```python
from build123d import *

# Parameters (mm, degrees)
SKETCH1_W                        = 72.8218
SKETCH1_H                        = 66.548
BOSS_EXTRUDE1_DEPTH              = 6.35
SKETCH2_R                        = 6.35
CUT_EXTRUDE1_DEPTH               = 7.35
SKETCH3_R                        = 2.12725
CUT_EXTRUDE2_DEPTH               = 7.35
SKETCH4_R                        = 2.12725
CUT_EXTRUDE3_DEPTH               = 7.35
SKETCH5_R                        = 2.12725
CUT_EXTRUDE4_DEPTH               = 7.35
SKETCH6_R                        = 3.4925
CUT_EXTRUDE5_DEPTH               = 4.572
F_1_8_0_125_DIAMETER_HOLE1_D     = 3.175
F_1_8_0_125_DIAMETER_HOLE1_DEPTH = 25.4
F_1_8_0_125_DIAMETER_HOLE1_TIP   = 0.953866233
CUT_EXTRUDE6_DEPTH               = 7.35
CUT_EXTRUDE7_DEPTH               = 7.35
CUT_EXTRUDE8_DEPTH               = 7.35
CUT_EXTRUDE9_DEPTH               = 7.35
CUT_EXTRUDE10_DEPTH              = 7.35


with BuildPart() as part:
    # Sketch1 → Boss-Extrude1 (new body)
    with BuildSketch(Plane.XY):
        with Locations((36.4109, 33.274)):
            Rectangle(SKETCH1_W, SKETCH1_H)
    extrude(amount=BOSS_EXTRUDE1_DEPTH)

    # Sketch2 → Cut-Extrude1 (cut, through all)
    with BuildSketch(Plane.XY.offset(6.35)):
        with Locations((59.1058, 46.482)):
            Circle(SKETCH2_R)
    extrude(amount=-CUT_EXTRUDE1_DEPTH, mode=Mode.SUBTRACT)

    # Sketch3 → Cut-Extrude2 (cut, through all)
    with BuildSketch(Plane.XY.offset(6.35)):
        with Locations((56.21655, 11.52525)):
            Circle(SKETCH3_R)
    extrude(amount=-CUT_EXTRUDE2_DEPTH, mode=Mode.SUBTRACT)

    # Sketch4 → Cut-Extrude3 (cut, through all)
    with BuildSketch(Plane.XY.offset(6.35)):
        with Locations((6.95325, 58.51525)):
            Circle(SKETCH4_R)
    extrude(amount=-CUT_EXTRUDE3_DEPTH, mode=Mode.SUBTRACT)

    # Sketch5 → Cut-Extrude4 (cut, through all)
    with BuildSketch(Plane.XY.offset(6.35)):
        with Locations((54.66715, 62.46495)):
            Circle(SKETCH5_R)
    extrude(amount=-CUT_EXTRUDE4_DEPTH, mode=Mode.SUBTRACT)

    # Sketch6 → Cut-Extrude5 (cut)
    with BuildSketch(Plane.XY.offset(6.35)):
        with Locations((54.66715, 62.46495)):
            Circle(SKETCH6_R)
    extrude(amount=-CUT_EXTRUDE5_DEPTH, mode=Mode.SUBTRACT)

    # 1/8 (0.125) Diameter Hole1
    with Locations(Plane.XY.offset(6.35)):
        with Locations((49.5808, 59.182), (68.6308, 59.109110049), (68.630660552, 33.70911005), (49.5808, 33.782)):
            Hole(F_1_8_0_125_DIAMETER_HOLE1_D / 2, depth=F_1_8_0_125_DIAMETER_HOLE1_DEPTH)
            with Locations((0, 0, -(F_1_8_0_125_DIAMETER_HOLE1_DEPTH + F_1_8_0_125_DIAMETER_HOLE1_TIP / 2))):  # 118° drill point
                Cone(0, F_1_8_0_125_DIAMETER_HOLE1_D / 2, F_1_8_0_125_DIAMETER_HOLE1_TIP, mode=Mode.SUBTRACT)

    # Sketch9 → Cut-Extrude6 (cut, through all)
    with BuildSketch(Plane.XY.offset(6.35)):
        Polygon((72.8218, 13.97), (58.8518, 0), (72.8218, 0), align=None)
    extrude(amount=-CUT_EXTRUDE6_DEPTH, mode=Mode.SUBTRACT)

    # Sketch10 → Cut-Extrude7 (cut, through all)
    with BuildSketch(Plane.XY.offset(6.35)):
        Polygon((3.683, 66.548), (0, 62.865), (0, 66.548), align=None)
    extrude(amount=-CUT_EXTRUDE7_DEPTH, mode=Mode.SUBTRACT)

    # Sketch11 → Cut-Extrude8 (cut, through all)
    with BuildSketch(Plane.XY.offset(6.35)):
        with BuildLine():
            Line((4.826, 53.831043168), (4.826, 0))
            Line((4.826, 0), (0, 0))
            Line((0, 0), (0, 57.192541634))
            ThreePointArc((0, 57.192541634), (3.109189127, 56.511289727), (4.826, 53.831043168))
        make_face()
    extrude(amount=-CUT_EXTRUDE8_DEPTH, mode=Mode.SUBTRACT)

    # Sketch12 → Cut-Extrude9 (cut, through all)
    with BuildSketch(Plane.XY.offset(6.35)):
        with BuildLine():
            Line((4.826, 29.972), (4.826, 0))
            Line((4.826, 0), (34.798, 0))
            ThreePointArc((34.798, 0), (13.604595554, 8.778595554), (4.826, 29.972))
        make_face()
    extrude(amount=-CUT_EXTRUDE9_DEPTH, mode=Mode.SUBTRACT)

    # Sketch13 → Cut-Extrude10 (cut, through all)
    with BuildSketch(Plane.XY.offset(6.35)):
        Polygon((69.7738, 66.548), (72.8218, 63.5), (72.8218, 66.548), align=None)
    extrude(amount=-CUT_EXTRUDE10_DEPTH, mode=Mode.SUBTRACT)


solid = part.part
```
For this review, take the finished solid that the model builds, in its own axes (mm). A direction names the side the tool comes from. Coordinates: 2 decimals unless noted, no trailing zeros. Loops run counter-clockwise (first coordinate to the right, second up) from the corner with the lowest first, then second, coordinate; pieces in that order, holes last. Notation, with made-up numbers: (56, 34.5) -> (115, 34.5) arc R10 ccw to (115, 50.5) -> close; hole circle Ø8 at (20, -21.5). An arc over 180 degrees is marked (long way). Return JSON: item names as keys, results as strings. Group by question number.
(1) Tool access review of faces 1 (the flat face through (4.826, 42, 3)), 2 (the flat face through (71.276, 65.045, 3.219)), 3 (the cylindrical face through (56.545, 65.41, 4.096)): name each direction out of +Z, -Z, +X, -X, +Y, -Y from which nothing blocks a thin tool from reaching the whole face with its end or side.
(2) Consider section D-D, the plane y = 5. Give the boundary of the cut face in (x, z).
(3) For pin 1 Ø3 at (y, z) = (39, 3.5) entering from -X; pin 2 Ø1 at (x, z) = (15.5, 4) entering from -Y; pin 3 Ø5 at (x, y) = (54.67, 62.46) entering from +Z, all flat-tipped, find the tip position at first contact; note any pin that passes through.
(4) Consider section C-C, the plane x = 8. Give the boundary of the cut face in (y, z).
(5) Consider section A-A, the plane x = 60. Give the boundary of the cut face in (y, z).
(6) Mouldability with a two-part tool opening along X and no side actions: class faces 4 (the flat face through (72.822, 38, 3)), 5 (the flat face through (36, 34, 6.35)), 6 (the flat face through (55, 60, 1.778)) as pulls with the +X half, pulls with the -X half, needs draft (parallel to the pull), parting line crosses it, or undercut.
(7) Consider section B-B, the plane z = 3. Count the separate pieces of the cut face and the enclosed holes in it, plus the area to 3 significant figures.
(8) To check wall thickness, follow L1, parallel to X at y = 60, z = 3.75; L2, parallel to X at y = 38, z = 0.5; L3, parallel to X at y = 11, z = 3.25. State the ranges of each line that lie inside material, in increasing order.
Results below:
{
 "1": {"face 1": "+Z, -Z, -X, -Y", "face 2": "+Z, -Z, +X, +Y", "face 3": "+Z"},
 "2": {"outline": "(18.22, 0) -> (63.85, 0) -> (63.85, 6.35) -> (18.22, 6.35) -> close"},
 "3": {"pin 1": "stops at x = 4.83", "pin 2": "stops at y = 6.63", "pin 3": "stops at z = 1.78"},
 "4": {"outline": "(16.55, 0) -> (56.66, 0) -> (56.66, 6.35) -> (16.55, 6.35) -> close; (60.37, 0) -> (66.55, 0) -> (66.55, 6.35) -> (60.37, 6.35) -> close"},
 "5": {"outline": "(1.15, 0) -> (40.2, 0) -> (40.2, 6.35) -> (1.15, 6.35) -> close; (52.77, 0) -> (66.55, 0) -> (66.55, 6.35) -> (52.77, 6.35) -> close"},
 "6": {"face 4": "pulls with the +X half", "face 5": "needs draft", "face 6": "undercut"},
 "7": {"separate pieces": "1", "enclosed holes": "8", "area": "4,050 mm2"},
 "8": {"L1": "x = 0 to 5.43, 8.48 to 48.22, 50.94 to 52.19, 57.14 to 67.32, 69.94 to 72.82", "L2": "x = 4.83 to 72.82", "L3": "x = 11.59 to 54.16, 58.28 to 69.85"}
}
